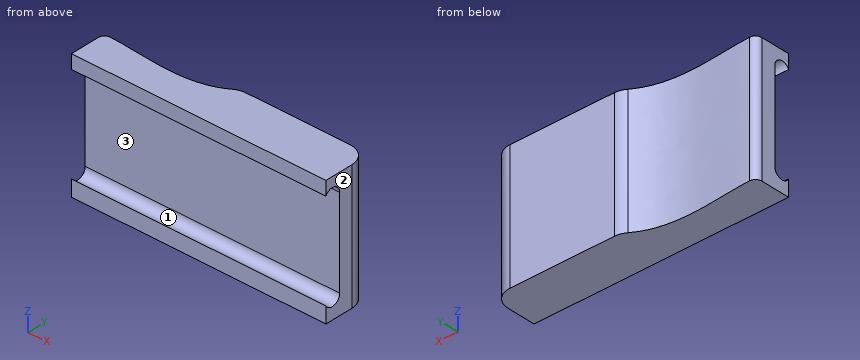
```python
from build123d import *

# Parameters (mm, degrees)
SKETCH1_W           = 400
SKETCH1_H           = 200
BOSS_EXTRUDE1_DEPTH = 60
CUT_EXTRUDE1_DEPTH  = 220
FILLET1_R           = 30
FILLET2_R           = 10
SKETCH9_W           = 400
SKETCH9_H           = 200
BOSS_EXTRUDE4_DEPTH = 15
CUT_EXTRUDE9_DEPTH  = 417.653333254


with BuildPart() as part:
    # Sketch1 → Boss-Extrude1 (new body)
    with BuildSketch(Plane(origin=(0, 0, 0), x_dir=(1, 0, 0), z_dir=(0, 1, 0))):
        Rectangle(SKETCH1_W, SKETCH1_H)
    extrude(amount=BOSS_EXTRUDE1_DEPTH)

    # Sketch3 → Cut-Extrude1 (cut)
    with BuildSketch(Plane.XY.offset(100)):
        with BuildLine():
            Line((-200, 41.033284164), (-200, 60))
            Line((-200, 60), (-3.947040737, 60))
            add(Edge.make_bspline(
                [(-200, 41.033284164), (-145.162329498, 43.56543882), (-56.826978114, 16.661467413), (-3.947040737, 60)],
                knots=[0, 0, 0, 0, 1, 1, 1, 1], degree=3))
        make_face()
    extrude(amount=-CUT_EXTRUDE1_DEPTH, mode=Mode.SUBTRACT)

    # Fillet1
    fillet1_edges = [part.edges().sort_by_distance(p)[0] for p in [
        (-3.947040737, 60, 0),
        (200, 60, 0),
    ]]
    fillet(fillet1_edges, radius=FILLET1_R)

    # Fillet2
    fillet2_edges = [part.edges().sort_by_distance(p)[0] for p in [
        (-200, 41.033284164, 0),
    ]]
    fillet(fillet2_edges, radius=FILLET2_R)

    # Sketch9 → Boss-Extrude4 (add)
    with BuildSketch(Plane.XZ):
        Rectangle(SKETCH9_W, SKETCH9_H)
    extrude(amount=BOSS_EXTRUDE4_DEPTH)

    # Sketch10 → Cut-Extrude9 (cut, through all)
    with BuildSketch(Plane.ZY.offset(200)):
        with BuildLine():
            Line((-74.762482239, -15), (1.674345002, -15))
            Line((1.674345002, -15), (1.674345002, 8.829888791))
            Line((1.674345002, 8.829888791), (-68.645654998, 8.829888791))
            ThreePointArc((-68.645654998, 8.829888791), (-80.94686607, -0.71254788), (-74.762482239, -15))
        make_face()
        with BuildLine():
            Line((1.674345002, 8.829888791), (1.674345002, -15))
            Line((1.674345002, -15), (78.111172243, -15))
            ThreePointArc((78.111172243, -15), (84.295556073, -0.71254788), (71.994345002, 8.829888791))
            Line((71.994345002, 8.829888791), (1.674345002, 8.829888791))
        make_face()
    extrude(amount=-CUT_EXTRUDE9_DEPTH, mode=Mode.SUBTRACT)


solid = part.part
```
The model under review builds one solid part; all positions refer to its coordinate system, in mm. Face numbers are marked on the shaded views. A direction names the side the tool comes from. Give positions to 0.01 mm unless a question says otherwise; leave off trailing zeros. Write each loop counter-clockwise with the first axis right and the second up, starting at its lowest first coordinate (ties: lowest second). Pieces come first, ordered by that corner, then holes.
(1) For P1, Ø6, axis at x = -2, z = 11.5, coming from the +Y side; P2, Ø8, axis at y = 30.5, z = 15.5, coming from the +X side; P3, Ø4, axis at x = -22, z = -4, coming from the +Y side; P4, Ø3, axis at x = 39, z = 70, coming from the -Y side, all flat-tipped, find the tip position at first contact; note any pin that passes through.
(2) Consider section B-B, the plane y = -1. Give the boundary of the cut face in (x, z), and give its area (3 significant figures).
(3) Tool access review of the marked faces 1, 2 and 3: name each direction out of +Z, -Z, +X, -X, +Y, -Y from which nothing blocks a thin tool from reaching the whole face with its end or side.
(4) To check wall thickness, follow L1, parallel to Y at x = 28, z = -19; L2, parallel to Z at x = 20, y = 2.5; L3, parallel to Y at x = -89.5, z = -46. State the ranges of each line that lie inside material, in increasing order.
(5) Consider section A-A, the plane x = 114. Give the boundary of the cut face in (y, z), and give its area (3 significant figures).
Returned:
1. P1: stops at y = 59.59
1. P2: stops at x = 200
1. P3: stops at y = 49.42
1. P4: stops at y = 8.83
2. outline: (-200, -100) - (200, -100) - (200, -81.02) - (-200, -81.02) - close; (-200, 84.37) - (200, 84.37) - (200, 100) - (-200, 100) - close
2. area: 13,800 mm2
3. face 1: +X, -X
3. face 2: +Z, -Z, +X, +Y, -Y
3. face 3: +X, -X, -Y
4. L1: y = 8.83 to 60
4. L2: z = -100 to -79.63, 82.98 to 100
4. L3: y = 8.83 to 35.09
5. outline: (-15, -100) - (60, -100) - (60, 100) - (-15, 100) - (-15, 78.11) arc R12.7 cw to (8.83, 71.99) - (8.83, -68.65) arc R12.7 cw to (-15, -74.76) - close
5. area: 11,200 mm2
